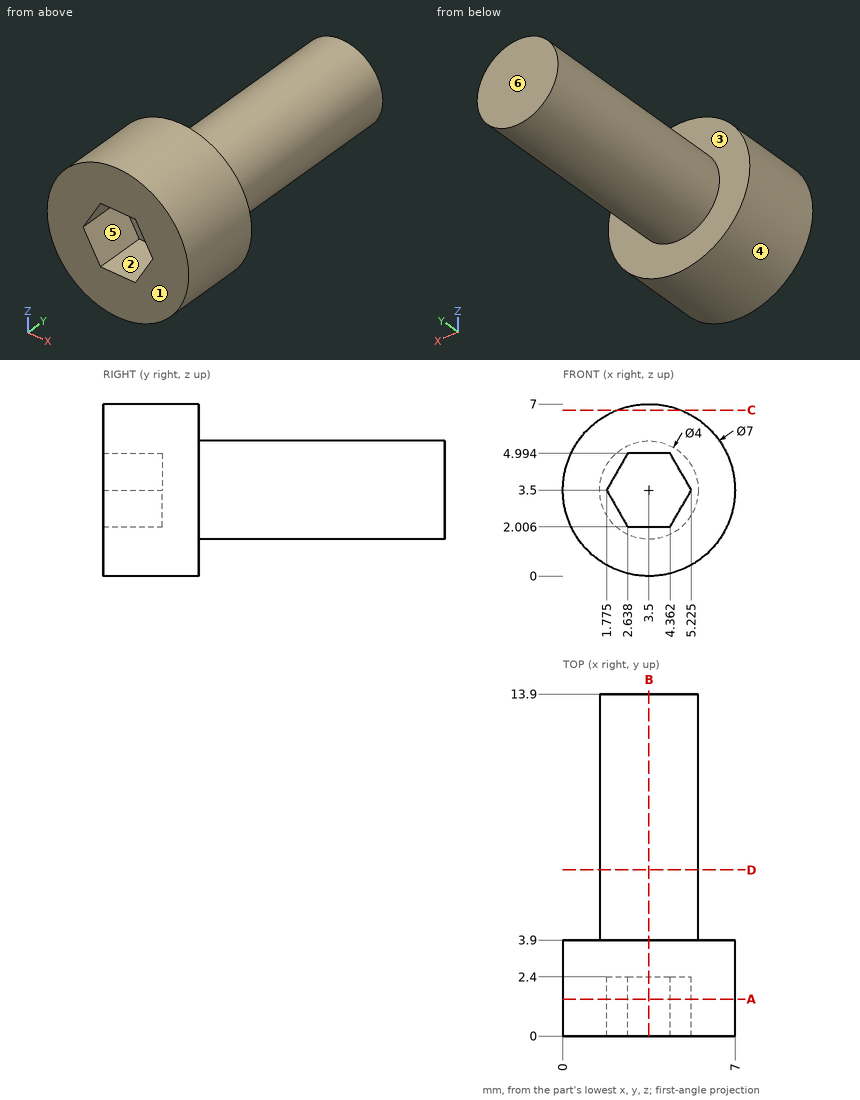
For this review, use the dimensioned drawing (mm, ordinates from the lowest corner) and the shaded views. A direction names the side the tool comes from. Give positions to 0.01 mm unless a question says otherwise; leave off trailing zeros. Order: outer loops, then holes, each group sorted by start corner. A loop starts at its lowest first (then second) coordinate and runs counter-clockwise, first axis right, second up. Notation, with made-up numbers: M 4.25,-26 L 22.25,-26 A37 cw 22.25,10 Z; hole C 26.5,-40 d10. An arc over 180 degrees is marked long. Use one line per item in the form item = value. Start each with the question number.
Item 1: We need section D-D on y = 6.75. Give the boundary of the cut face in (x, z).
Item 2: Insertion check: pin 1 Ø2 at (x, y) = (3, 7.5) entering from +Z; pin 2 Ø3 at (y, z) = (11, 3) entering from +X. Each pin has a flat end and moves straight along its axis. Give the tip position at first contact, or say it passes through.
Item 3: We need section A-A on y = 1.5. Give the boundary of the cut face in (x, z) (1 decimal).
Item 4: For the marked faces 1, 2 and 3, list the 3-axis set-ups (+Z, -Z, +X, -X, +Y, -Y) from which the entire face can be reached by the end or side of a thin tool; tool diameter is ignored.
Item 5: The part is to be moulded in two halves that separate along X. For the marked faces 4, 5 and 6, say which applies: pulls with the +X half, pulls with the -X half, needs draft (parallel to the pull), parting line crosses it, or undercut.
Item 6: To check wall thickness, follow line 1 along Y through (x, z) = (6.25, 1.75); line 2 along X through (y, z) = (5.5, 3.5); line 3 along X through (y, z) = (0.75, 4.25). State the ranges of each line that lie inside material, in increasing order. Write a range as from..to.
Item 7: We need section C-C on z = 6.75. Give the boundary of the cut face in (x, y), plus the area to 3 significant figures.
Item 8: We need section B-B on x = 3.5. Give the boundary of the cut face in (y, z).
Completed:
q1.outline = C 3.5,3.5 d4
q2.pin_1 = 5.5
q2.pin_2 = 5.5
q3.outline = C 3.5,3.5 d7; hole M 1.8,3.5 L 2.6,2 L 4.4,2 L 5.2,3.5 L 4.4,5 L 2.6,5 Z
q4.face_1 = +Z, -Z, +X, -X, -Y
q4.face_2 = -Y
q4.face_3 = +Y
q5.face_4 = parting line crosses it
q5.face_5 = undercut
q5.face_6 = needs draft
q6.line_1 = 0..3.9
q6.line_2 = 1.5..5.5
q6.line_3 = 0.08..2.21, 4.79..6.92
q7.outline = M 2.2,0 L 4.8,0 L 4.8,3.9 L 2.2,3.9 Z
q7.area = 10.1 mm²
q8.outline = M 0,0 L 3.9,0 L 3.9,1.5 L 13.9,1.5 L 13.9,5.5 L 3.9,5.5 L 3.9,7 L 0,7 L 0,4.99 L 2.4,4.99 L 2.4,2.01 L 0,2.01 Z
